Read the model definition and answer for the solid it produces. Units are mm, in the model's axes. A direction names the side the tool comes from. Round coordinates to 2 decimals unless told otherwise and drop trailing zeros. Order: outer loops, then holes, each group sorted by start corner. A loop starts at its lowest first (then second) coordinate and runs counter-clockwise, first axis right, second up. Notation, with made-up numbers: (12.5, -23) - (40.5, -23) arc R24 ccw to (40.5, 11) - close; hole circle Ø11 at (31.25, 87.5). An arc over 180 degrees is marked (long way). Answer as a JSON object with one key per item and string values. Group by question number.
Q1. The mould has two halves that part along Y. Classify faces 5 (the flat face through (0, -18, -8)), 6 (the flat face through (-30, 44, 0)), 7 (the flat face through (0, 69, 0)): pulls with the +Y half, pulls with the -Y half, needs draft (parallel to the pull), parting line crosses it, or undercut.
Q2. A tool of negligible diameter and unlimited length cuts with its end or side. For faces 1 (the flat face through (-24, 60, -15)), 2 (the flat face through (0, 71, 12)), 3 (the flat face through (0, 21, 0)), 4 (the flat face through (0, 0, 0)), from which of +Z, -Z, +X, -X, +Y, -Y can it reach the whole face along a straight path? Write none if from no direction.
Q3. A cutting plane is placed at A-A on y = 51.5. Determine the outline of the cut face in (x, z).
Q4. A cutting plane is placed at C-C on z = 0. Determine the outline of the cut face in (x, y), and give its area (3 significant figures).
Q5. A cutting plane is placed at B-B on x = 21. Determine the outline of the cut face in (y, z).
Q6. Consider line 1 (X direction, y = 37.5, z = -13); line 2 (Z direction, x = 0, y = -9.25); line 3 (Y direction, x = -4.5, z = 15). Determine where each line is inside the solid, lowest interval first.
Q7. Given pin 1 Ø5 at (x, z) = (-14, -16.5) entering from -Y; pin 2 Ø9 at (x, y) = (2, 69) entering from -Z; pin 3 Ø5.5 at (x, y) = (2, 67.5) entering from +Z, each flat-ended and moving along its own axis, determine where each tip first touches the part or whether it passes through.
Autodesk Fusion 360 part; units mm, degrees
sketch "Sketch1" plane through (0, 0, 0) normal (0, 1, 0) x (1, 0, 0)
  line L0 (30, 18) -> (-30, 18)
  line L1 (-30, 18) -> (-30, -18)
  line L2 (-30, -18) -> (30, -18)
  line L3 (30, -18) -> (30, 18)
extrude "Extrude1" add sketch "Sketch1" along normal blind 90
sketch "Sketch2" plane through (0, 0, 0) normal (0, -1, 0) x (1, 0, 0)
  line L0 (30, -18) -> (30, 18)
  line L1 (30, 18) -> (-30, 18)
  line L2 (-30, 18) -> (-30, -18)
  line L3 (-30, -18) -> (30, -18)
  circle A0 centre (0, 0) radius 18
  circle A1 centre (0, 0) radius 6
  dimension "d5" = 12
extrude "Extrude2" add sketch "Sketch2" along normal blind 18 contours A0
thread "Thread1" thread offset 0 thread length 10
sketch "Sketch3" plane through (-30, 0, 0) normal (-1, 0, 0) x (0, -1, 0)
  line L0 (0, -18) -> (0, 18)
  line L1 (0, 18) -> (-90, 18)
  line L2 (-90, 18) -> (-90, -18)
  line L3 (-90, -18) -> (0, -18)
  line L4 (-78, -18) -> (-60, -18)
  line L5 (-60, -18) -> (-60, -12)
  line L6 (-60, -12) -> (-78, -12)
  line L7 (-78, -12) -> (-78, -18)
extrude "Extrude3" cut sketch "Sketch3" against normal blind 60 contours L3 L4 L5 L6 L7
sketch "Sketch4" plane through (-30, 0, 0) normal (-1, 0, 0) x (0, -1, 0)
  line L0 (-78, -18) -> (-78, -12)
  line L1 (-78, -12) -> (-60, -12)
  line L2 (-60, -12) -> (-60, -18)
  line L3 (-60, -18) -> (0, -18)
  line L4 (0, -18) -> (0, 18)
  line L5 (0, 18) -> (-90, 18)
  line L6 (-90, 18) -> (-90, -18)
  line L7 (-90, -18) -> (-78, -18)
  line L8 (-78, 18) -> (-60, 18)
  line L9 (-60, 18) -> (-60, 12)
  line L10 (-60, 12) -> (-78, 12)
  line L11 (-78, 12) -> (-78, 18)
extrude "Extrude4" cut sketch "Sketch4" against normal blind 60 contours L5 L8 L9 L10 L11
sketch "Sketch5" plane through (0, 0, 18) normal (0, 0, 1) x (-1, 0, 0)
  line L0 (-30, -60) -> (30, -60)
  line L1 (30, -60) -> (30, 0)
  line L2 (30, 0) -> (0, 0)
  line L3 (0, 0) -> (-30, 0)
  line L4 (-30, 0) -> (-30, -60)
  line L5 (-30, 0) -> (-30, -21)
  line L6 (-18, -21) -> (-18, -69)
  line L7 (-18, -69) -> (18, -69)
  line L8 (18, -69) -> (18, -21)
  line L9 (18, -21) -> (-18, -21)
  dimension "d21" = 12
  dimension "d22" = 48
  dimension "d23" = 36
extrude "Extrude5" cut sketch "Sketch5" against normal blind 36 contours L0 L6 L8 L9 | L0 L6 L7 L8
Result set:
{
 "1": {"face 5": "pulls with the -Y half", "face 6": "needs draft", "face 7": "undercut"},
 "2": {"face 1": "-Z, +X, -X", "face 2": "+Z, +X, -X", "face 3": "+Z, -Z", "face 4": "-Y"},
 "3": {"outline": "(-30, -18) - (-18, -18) - (-18, 18) - (-30, 18) - close; (18, -18) - (30, -18) - (30, 18) - (18, 18) - close"},
 "4": {"outline": "(-30, 0) - (-18, 0) - (-18, -18) - (-6, -18) - (-6, 0) - (6, 0) - (6, -18) - (18, -18) - (18, 0) - (30, 0) - (30, 90) - (-30, 90) - close; hole (-18, 21) - (18, 21) - (18, 69) - (-18, 69) - close", "area": "4,100 mm²"},
 "5": {"outline": "(0, -18) - (60, -18) - (60, -12) - (78, -12) - (78, -18) - (90, -18) - (90, 18) - (78, 18) - (78, 12) - (60, 12) - (60, 18) - (0, 18) - close"},
 "6": {"line 1": "x = -30 to -18, 18 to 30", "line 2": "z = -18 to -6, 6 to 18", "line 3": "y = -18 to 21, 78 to 90"},
 "7": {"pin 1": "stops at y = 0", "pin 2": "stops at z = -12", "pin 3": "stops at z = 12"}
}
